Could you check a few things on this model? Use its own coordinates, in mm. Face numbers are marked on the shaded views. A direction names the side the tool comes from. Coordinates: 2 decimals unless noted, no trailing zeros. Loops run counter-clockwise (first coordinate to the right, second up) from the corner with the lowest first, then second, coordinate; pieces in that order, holes last. Notation, with made-up numbers: M -34.5,58 L -25.5,58 A34 ccw -25.5,89 Z; hole C 12,59 d9. An arc over 180 degrees is marked long. Write each question's results on one line, items separated by ' | '.
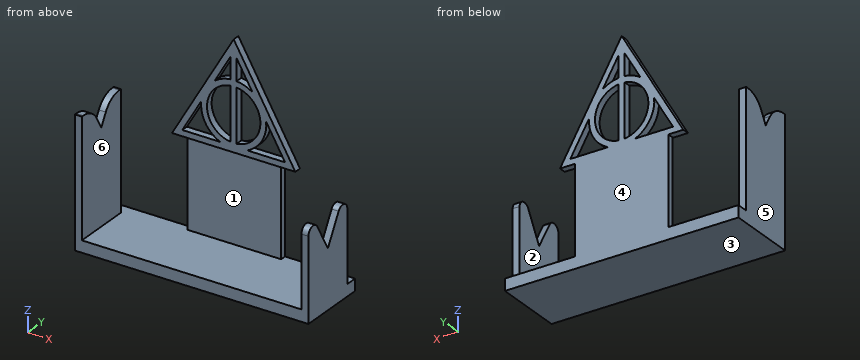
```python
from build123d import *

# Parameters (mm, degrees)
F1_DEPTH  = 3
F2_W      = 20
F2_H      = 40
F3_DEPTH  = 2.5
F5_DEPTH  = 30
F6_W      = 3
F6_H      = 25
F7_DEPTH  = 50
F9_DEPTH  = 25
F11_DEPTH = 10
F12_R     = 10
F13_R     = 3


with BuildPart() as f1:
    # F0 (on Front) → F1 (new body)
    with BuildSketch(Plane.XZ):
        Polygon((-26.3964543073, -2.54), (26.3964543073, -2.54), (0, 43.18), align=None)
        with BuildLine():
            Line((-5.8198711326, 0), (-21.9970452561, 0))
            Line((-21.9970452561, 0), (-13.9084581944, 14.0098437524))
            ThreePointArc((-13.9084581944, 14.0098437524), (-12.0983748909, 5.715), (-5.8198711326, 0))
        make_face(mode=Mode.SUBTRACT)
        with BuildLine():
            ThreePointArc((-1.27, 1.3407746743), (-11.43, 12.7), (-1.27, 24.0592253257))
            Line((-1.27, 24.0592253257), (-1.27, 1.3407746743))
        make_face(mode=Mode.SUBTRACT)
        with BuildLine():
            Line((13.9084581944, 14.0098437524), (21.9970452561, 0))
            Line((21.9970452561, 0), (5.8198711326, 0))
            ThreePointArc((5.8198711326, 0), (12.0983748909, 5.715), (13.9084581944, 14.0098437524))
        make_face(mode=Mode.SUBTRACT)
        with BuildLine():
            Line((1.27, 1.3407746743), (1.27, 24.0592253257))
            ThreePointArc((1.27, 24.0592253257), (11.43, 12.7), (1.27, 1.3407746743))
        make_face(mode=Mode.SUBTRACT)
        with BuildLine():
            Line((-8.0885870618, 24.0901562476), (-1.27, 35.9002954744))
            Line((-1.27, 35.9002954744), (-1.27, 26.6121529606))
            ThreePointArc((-1.27, 26.6121529606), (-4.8462258308, 25.8024804979), (-8.0885870618, 24.0901562476))
        make_face(mode=Mode.SUBTRACT)
        with BuildLine():
            Line((1.27, 26.6121529606), (1.27, 35.9002954744))
            Line((1.27, 35.9002954744), (8.0885870618, 24.0901562476))
            ThreePointArc((8.0885870618, 24.0901562476), (4.8462258308, 25.8024804979), (1.27, 26.6121529606))
        make_face(mode=Mode.SUBTRACT)
    extrude(amount=F1_DEPTH)

    # F2 (on Front) → F3 (join)
    with BuildSketch(Plane.XZ):
        with Locations((-10, -20)):
            Rectangle(F2_W, F2_H)
        with Locations((10, -20)):
            Rectangle(F2_W, F2_H)
    extrude(amount=F3_DEPTH)

    # F4 (on Front) → F5 (join)
    with BuildSketch(Plane.XZ):
        Polygon((20, -40), (-20, -40), (-50, -40), (-50, -45), (50, -45), (50, -40), align=None)
    extrude(amount=F5_DEPTH)

    # F6 (on face) → F7 (join)
    with BuildSketch(Plane.XY.offset(-40)):
        with Locations((-48.5, -17.5)):
            Rectangle(F6_W, F6_H)
        with Locations((48.5, -17.5)):
            Rectangle(F6_W, F6_H)
    extrude(amount=F7_DEPTH)

    # F8 (on face) → F9 (cut)
    with BuildSketch(Plane(origin=(-50, 0, 0), x_dir=(0, -1, 0), z_dir=(-1, 0, 0))):
        Polygon((23.2735026919, 10), (11.7264973081, 10), (17.5, 0), align=None)
    extrude(amount=-F9_DEPTH, mode=Mode.SUBTRACT)

    # F10 (on face) → F11 (cut)
    with BuildSketch(Plane.YZ.offset(50)):
        Polygon((-17.5, 10), (-34.8205080757, 10), (-17.5, -20), align=None)
        Polygon((-17.5, 10), (-17.5, -20), (-0.1794919243, 10), align=None)
    extrude(amount=-F11_DEPTH, mode=Mode.SUBTRACT)

    # F12
    f12_edges = [f1.edges().sort_by_distance(p)[0] for p in [
        (-48.5, -11.726497, 10),
        (-48.5, -23.273503, 10),
    ]]
    fillet(f12_edges, radius=F12_R)

    # F13
    f13_edges = [f1.edges().sort_by_distance(p)[0] for p in [
        (48.5, -30, 1.650635),
        (48.5, -5, 1.650635),
    ]]
    fillet(f13_edges, radius=F13_R)


solid = f1.part
```
(1) Please list where these lines run through material, in increasing order: probe 1 along X at (y, z) = (-26.5, -9); probe 2 along Z at (x, y) = (5, -1.5); probe 3 along Z at (x, y) = (36, -3.5). Write a range as from..to.
Reported:
probe 1: x = -50..-47, 47..50 | probe 2: z = -45..2.42, 22.98..25.74, 29.44..34.52 | probe 3: z = -45..-40
(2) Imagine slicing it at A-A, the plane z = -38.5. List the corners of the cut face in (x, y) for me, and give its area (3 significant figures).
Reported:
outline: M -50,-30 L -47,-30 L -47,-5 L -50,-5 Z; M -20,-2.5 L 20,-2.5 L 20,0 L -20,0 Z; M 47,-30 L 50,-30 L 50,-5 L 47,-5 Z | area: 250 mm2
(3) Will these pins go through, and if not, where does the flat tip stop? P1, Ø3, axis at y = -8, z = 8, coming from the +X side; P2, Ø4, axis at x = 13.5, y = -21.5, coming from the +Z side; P3, Ø0.9, axis at y = -1.5, z = 10.5, coming from the +X side.
Reported:
P1: stops at x = -47 | P2: stops at z = -40 | P3: stops at x = 19.13
(4) Which directions (+Z, -Z, +X, -X, +Y, -Y) give clear straight access to the entire face, cutting with the end or side of a thin tool? Please do the marked faces 1, 2 and 3.
Reported:
face 1: +X, -X, -Y | face 2: +Z, +Y, -Y | face 3: -Z, +X, -X, +Y, -Y
(5) Imagine slicing it at C-C, the plane z = -5. List the corners of the cut face in (x, y) for me, and give its area (3 significant figures).
Reported:
outline: M -50,-30 L -47,-30 L -47,-5 L -50,-5 Z; M -20,-2.5 L 20,-2.5 L 20,0 L -20,0 Z | area: 175 mm2
(6) Imagine slicing it at B-B, the plane z = 7.5. List the corners of the cut face in (x, y) for me.
Reported:
outline: M -50,-30 L -47,-30 L -47,-22.43 L -50,-22.43 Z; M -50,-12.57 L -47,-12.57 L -47,-5 L -50,-5 Z; M -20.6,-3 L -17.67,-3 L -17.67,0 L -20.6,0 Z; M -12.97,-3 L -10.18,-3 L -10.18,0 L -12.97,0 Z; M -1.27,-3 L 1.27,-3 L 1.27,0 L -1.27,0 Z; M 10.18,-3 L 12.97,-3 L 12.97,0 L 10.18,0 Z; M 17.67,-3 L 20.6,-3 L 20.6,0 L 17.67,0 Z
(7) Imagine slicing it at D-D, the plane y = -7.5. List the corners of the cut face in (x, z) for me, and give its area (3 significant figures).
Reported:
outline: M -50,-45 L 50,-45 L 50,-6.59 L 47,-6.59 L 47,-40 L -47,-40 L -47,9.88 L -50,9.88 Z | area: 750 mm2
(8) If we mould it in two halves opening along X, with no side actions, what happens to the marked faces 4, 5 and 6? For each: released by +X, released by -X, zero draft, split by the parting line, or undercut.
Reported:
face 4: zero draft | face 5: released by -X | face 6: undercut
